from build123d import *

# Parameters (mm, degrees)
BOSS_EXTRUDE1_DEPTH     = 6
SHELL1_T                = 2
BOSS_EXTRUDE2_DEPTH     = 12
CUT_EXTRUDE1_DEPTH      = 105.548062061
CUT_EXTRUDE1_DEPTH_BACK = 105.548062061
SKETCH4_OUTSIDE_W       = 127.703
SKETCH4_OUTSIDE_H       = 47.702
SKETCH4_OUTSIDE_R       = 5
BOSS_EXTRUDE3_START     = -3
SKETCH5_R               = 5
BOSS_EXTRUDE3_DEPTH     = 3
SKETCH8_W               = 2
SKETCH8_H               = 3
CUT_EXTRUDE2_DEPTH      = 20.507580381


with BuildPart() as part:
    # Sketch1 → Boss-Extrude1 (new, symmetric)
    with BuildSketch(Plane.XY):
        with BuildLine():
            add(Edge.make_bspline(
                [(0, 0), (-0.020523105, 1.211959263), (0.67437266, 2.857215342), (1.905623999, 4.78389108), (3.228212227, 6.302382051), (4.893886607, 7.740810658), (7.226107258, 9.264300756), (10.552653396, 10.717178582), (14.932037071, 11.831530653), (19.991297272, 12.255898832), (25.003683181, 12.218808276), (31.681712165, 11.857586647), (40.030453626, 10.974271434), (50.024814986, 9.447886993), (60.008390595, 7.611152922), (69.999350586, 5.696721586), (83.333766276, 3.168852276), (93.333116862, 1.265573862), (100, 0)],
                knots=[0, 0, 0, 0, 0.032626759, 0.049882871, 0.06427589, 0.089250813, 0.111667998, 0.142584384, 0.191135501, 0.238340392, 0.285329255, 0.332381604, 0.426846937, 0.521876031, 0.61736406, 0.713023045, 0.80868203, 1, 1, 1, 1], degree=3))
            add(Edge.make_bspline(
                [(0, 0), (0.036655271, -0.696109017), (0.772960092, -1.382467179), (1.96178056, -1.978761756), (3.324506087, -2.315299728), (4.988662397, -2.651222943), (7.325816413, -2.960951495), (10.662744647, -3.183232196), (14.999725999, -3.252330394), (19.999719582, -3.317988032), (25.00025256, -3.335705262), (31.666881467, -3.233674), (40.002372591, -3.118326111), (50.001627017, -2.749659581), (60.002529003, -2.322582922), (69.997554247, -1.759547439), (83.37248003, -1.331343132), (93.243437862, 0.963839901), (100, 0)],
                knots=[0, 0, 0, 0, 0.017855622, 0.028908701, 0.039175102, 0.059339021, 0.079290733, 0.109028899, 0.158476478, 0.20791091, 0.257341883, 0.306776316, 0.405654078, 0.504572951, 0.603530351, 0.702515599, 0.801543493, 1, 1, 1, 1], degree=3))
        make_face()
    extrude(amount=BOSS_EXTRUDE1_DEPTH, both=True)

    # Shell1
    shell1_openings = [part.faces().sort_by_distance(p)[0] for p in [
        (38.486858992, 3.393824358, 6),
        (38.486858992, 3.393824358, -6),
    ]]
    offset(amount=SHELL1_T, openings=shell1_openings)

    # Sketch3 → Boss-Extrude2 (add)
    with BuildSketch(Plane.XY.offset(6)):
        with BuildLine():
            add(Edge.make_bspline(
                [(0, 0), (0.036655271, -0.696109017), (0.772960092, -1.382467179), (1.96178056, -1.978761756), (3.324506087, -2.315299728), (4.988662397, -2.651222943), (7.325816413, -2.960951495), (10.662744647, -3.183232196), (14.999725999, -3.252330394), (19.999719582, -3.317988032), (25.00025256, -3.335705262), (31.666881467, -3.233674), (40.002372591, -3.118326111), (50.001627017, -2.749659581), (60.002529003, -2.322582922), (69.997554247, -1.759547439), (83.37248003, -1.331343132), (93.243437862, 0.963839901), (100, 0)],
                knots=[0, 0, 0, 0, 0.017855622, 0.028908701, 0.039175102, 0.059339021, 0.079290733, 0.109028899, 0.158476478, 0.20791091, 0.257341883, 0.306776316, 0.405654078, 0.504572951, 0.603530351, 0.702515599, 0.801543493, 1, 1, 1, 1], degree=3))
            add(Edge.make_bspline(
                [(100, 0), (93.333116862, 1.265573862), (83.333766276, 3.168852276), (69.999350586, 5.696721586), (60.008390595, 7.611152922), (50.024814986, 9.447886993), (40.030453626, 10.974271434), (31.681712165, 11.857586647), (25.003683181, 12.218808276), (19.991297272, 12.255898832), (14.932037071, 11.831530653), (10.552653396, 10.717178582), (7.226107258, 9.264300756), (4.893886607, 7.740810658), (3.228212227, 6.302382051), (1.905623999, 4.78389108), (0.67437266, 2.857215342), (-0.020523105, 1.211959263), (0, 0)],
                knots=[0, 0, 0, 0, 0.19131797, 0.286976955, 0.38263594, 0.478123969, 0.573153063, 0.667618396, 0.714670745, 0.761659608, 0.808864499, 0.857415616, 0.888332002, 0.910749187, 0.93572411, 0.950117129, 0.967373241, 1, 1, 1, 1], degree=3))
        make_face()
    extrude(amount=BOSS_EXTRUDE2_DEPTH)

    # Sketch4 outside → Cut-Extrude1 (cut, two sides: drawn at the far end of the back side and taken through both)
    with BuildSketch(Plane(origin=(0, 0, 0), x_dir=(1, 0, 0), z_dir=(0, 1, 0)).offset(-CUT_EXTRUDE1_DEPTH_BACK)):
        with Locations((49.9995, -6)):
            Rectangle(SKETCH4_OUTSIDE_W, SKETCH4_OUTSIDE_H)
        with Locations(Location((62.007047228, -12, 0), (0, 0, 270))):
            Circle(SKETCH4_OUTSIDE_R, mode=Mode.SUBTRACT)
    extrude(amount=CUT_EXTRUDE1_DEPTH + CUT_EXTRUDE1_DEPTH_BACK, mode=Mode.SUBTRACT)

    # Sketch5 → Boss-Extrude3 (add)
    with BuildSketch(Plane(origin=(0, 0, 0), x_dir=(1, 0, 0), z_dir=(0, 1, 0)).offset(BOSS_EXTRUDE3_START)):
        with Locations(Location((62.007047228, -12, 0), (0, 0, 270))):
            Circle(SKETCH5_R)
    extrude(amount=BOSS_EXTRUDE3_DEPTH)

    # Sketch6 → Cut-Revolve3 (revolve, cut)
    with BuildSketch(Plane(origin=(62.007047228, 0, 0), x_dir=(0, 0, -1), z_dir=(1, 0, 0))):
        Polygon((-12, 2), (-12, -3), (-10.5, -3), (-10.5, 0), (-9, 0), (-9, 2), align=None)
    revolve(axis=Axis((62.007047228, 2, 12), (0, -1, 0)), mode=Mode.SUBTRACT)

    # Sketch8 → Cut-Extrude2 (cut, through all)
    with BuildSketch(Plane(origin=(62.007047228, 0, 0), x_dir=(0, 0, -1), z_dir=(1, 0, 0))):
        Polygon((-15, 0), (-13, 0), (-11, 0), (-9, 0), (-9, 2), (-15, 2), align=None)
        with Locations((-12, -1.5)):
            Rectangle(SKETCH8_W, SKETCH8_H)
    extrude(amount=CUT_EXTRUDE2_DEPTH, mode=Mode.SUBTRACT)


solid = part.part
Check sheet for the modelled part. Datum: model origin and axes. Units: mm. A direction names the side the tool comes from. Round coordinates to 2 decimals unless told otherwise and drop trailing zeros. Order: outer loops, then holes, each group sorted by start corner. A loop starts at its lowest first (then second) coordinate and runs counter-clockwise, first axis right, second up.
Q1. Cross-section at C-C, the plane y = -0.5. Enter the section's corners in (x, z).
Filled sheet:
outline: (63.13, 11) arc R1.5 cw (long way) to (63.13, 13) - (66.91, 13) arc R5 ccw (long way) to (66.91, 11) - close
Q2. Cross-section at B-B, the plane x = 66.5. Give the number of separate pieces and of enclosed holes in the cut face, plus the area to 3 significant figures.
Filled sheet:
separate pieces: 3
enclosed holes: 0
area: 26.3 mm2
Q3. Set-up check for faces 4 (the face through (65, -2, 11)), 5 (the face through (60.508, -1.479, 12.051)), 6 (the face through (64, 1, 9)): record each of +Z, -Z, +X, -X, +Y, -Y from which the full face is reachable in a straight line by a thin tool's end or side.
Filled sheet:
face 4: +X, -Y
face 5: -Y
face 6: +X
Q4. Draft check along Y on faces 1 (the face through (59.008, 1.014, 12.066)), 2 (the face through (65, -2, 13)), 3 (the face through (60, -3, 12)). Enter one of: pulls with the +Y half, pulls with the -Y half, needs draft (parallel to the pull), parting line crosses it, or undercut.
Filled sheet:
face 1: undercut
face 2: needs draft
face 3: pulls with the -Y half
Q5. Depth check by flat-ended pin: P1, Ø1.5, axis at x = 58.5, y = 6.5, coming from the -Z side; P2, Ø3, axis at x = 60.5, z = 12.5, coming from the +Y side; P3, Ø2, axis at x = 63.5, y = 1.5, coming from the +Z side. Enter the tip coordinate at first touch or a pass-through.
Filled sheet:
P1: stops at z = 7.83
P2: stops at y = 7.79
P3: stops at z = 16.98
Q6. Scan lines: L1, parallel to Y at x = 62.25, z = 14.25; L2, parallel to Y at x = 65.5, z = 14; L3, parallel to Z at x = 61.5, y = 0.75. Record each from-to range of solid material in increasing order.
Filled sheet:
L1: y = -3 to 0, 2 to 7.18
L2: y = -3 to 0, 2 to 6.56
L3: z = 7.03 to 9.04, 14.96 to 16.97
Q7. Cross-section at A-A, the plane y = 2.25. Enter the section's corners in (x, z), plus the area to 3 significant figures.
Filled sheet:
outline: circle Ø10 at (62.01, 12)
area: 78.5 mm2
